CAD build for the part. Positions are in the model's coordinates, mm. A direction names the side the tool comes from. Give positions to 0.01 mm unless a question says otherwise; leave off trailing zeros. Order: outer loops, then holes, each group sorted by start corner. A loop starts at its lowest first (then second) coordinate and runs counter-clockwise, first axis right, second up. Notation, with made-up numbers: M -34.5,74.5 L -3.5,74.5 A19 ccw -3.5,107.5 Z; hole C 12,-17 d6. An arc over 180 degrees is marked long. Put each result on its own line as item: value. Start each with the question number.
1) Cut at B-B (x = -49). Write the cut outline in (y, z).
2) Cut at A-A (y = 15.5). Write the cut outline in (x, z), and give its area (3 significant figures).
3) Two-plate mould, pull along Y, no slides. Class faces 1 (the face through (-51.5, 0, 1)), 2 (the face through (-49.921, 16.345, 0.862)), 3 (the face through (11, -13.99, 5)): released by +Y, released by -Y, zero draft, split by the parting line, or undercut.
4) Tool access for faces 4 (the face through (49, 0, 4.2)), 5 (the face through (49.523, -5.072, 2.932)), 6 (the face through (49.47, 4.92, 2.93)), 7 (the face through (-23.96, -1, 5)), 8 (the face through (11, 13.01, 5)): list every direction of +Z, -Z, +X, -X, +Y, -Y with a clear straight run to the whole face (end or side of a thin tool).
5) Pin check, flat tips, straight feed: pin 1 (1.2 mm diameter, centred on x = 50, y = -1.5, fed in from +Z); pin 2 (1 mm diameter, centred on y = -14, z = 4.5, fed in from -X); pin 3 (1.5 mm diameter, centred on x = -11.5, z = 7, fed in from -Y). Stop position of each tip, or through.
6) Cut at C-C (x = -18). Write the cut outline in (y, z).
7) Drill centre lines: line 1 (Y direction, x = 49, z = 1.3); line 2 (Z direction, x = -24.5, y = 12); line 3 (Y direction, x = 1.5, z = 8.25). Where is each one in solid material? Low to high. Write a range as [from, to].
8) Cut at D-D (y = 10). Write the cut outline in (x, z), and give its area (3 significant figures).
```python
from build123d import *

# Parameters (mm, degrees)
CROQUIS1_W              = 103
CROQUIS1_H              = 36
SALIENTE_EXTRUIR1_DEPTH = 1.7
CROQUIS2_W              = 71.45
CROQUIS2_H              = 27
SALIENTE_EXTRUIR2_DEPTH = 7.05
CROQUIS3_R              = 1.25
CORTAR_EXTRUIR1_DEPTH   = 6
SALIENTE_EXTRUIR3_DEPTH = 2.5


with BuildPart() as part:
    # Croquis1 → Saliente-Extruir1 (new body)
    with BuildSketch(Plane.XY):
        Rectangle(CROQUIS1_W, CROQUIS1_H)
    extrude(amount=SALIENTE_EXTRUIR1_DEPTH)

    # Croquis2 → Saliente-Extruir2 (add)
    with BuildSketch(Plane.XY.offset(1.7)):
        with Locations((11.765, -0.49)):
            Rectangle(CROQUIS2_W, CROQUIS2_H)
    extrude(amount=SALIENTE_EXTRUIR2_DEPTH)

    # Croquis3 → Cortar-Extruir1 (cut)
    with BuildSketch(Plane.XY.offset(1.7)):
        with Locations((-49, 15.5)):
            Circle(CROQUIS3_R)
        with Locations((-49, -15.5)):
            Circle(CROQUIS3_R)
        with Locations((49, 15.5)):
            Circle(CROQUIS3_R)
        with Locations((49, -15.5)):
            Circle(CROQUIS3_R)
    extrude(amount=-CORTAR_EXTRUIR1_DEPTH, mode=Mode.SUBTRACT)

    # Croquis4 → Saliente-Extruir3 (add)
    with BuildSketch(Plane.XY.offset(1.7)):
        Polygon((47.49, 7.01), (51.5, 2.775802991), (51.5, -2.234197009), (47.49, -7.99), align=None)
    extrude(amount=SALIENTE_EXTRUIR3_DEPTH)


solid = part.part
```
Solution:
1. outline: M -18,0 L -16.75,0 L -16.75,1.7 L -18,1.7 Z; M -14.25,0 L 14.25,0 L 14.25,1.7 L -14.25,1.7 Z; M 16.75,0 L 18,0 L 18,1.7 L 16.75,1.7 Z
2. outline: M -51.5,0 L -50.25,0 L -50.25,1.7 L -51.5,1.7 Z; M -47.75,0 L 47.75,0 L 47.75,1.7 L -47.75,1.7 Z; M 50.25,0 L 51.5,0 L 51.5,1.7 L 50.25,1.7 Z
2. area: 167 mm²
3. face 1: zero draft
3. face 2: undercut
3. face 3: released by -Y
4. face 4: +Z, +X, +Y, -Y
4. face 5: +Z, +X, -Y
4. face 6: +Z, +X, +Y
4. face 7: +Z, -X, +Y, -Y
4. face 8: +Z, +X, -X, +Y
5. pin 1: z = 4.2
5. pin 2: x = -23.96
5. pin 3: y = -13.99
6. outline: M -18,0 L 18,0 L 18,1.7 L 13.01,1.7 L 13.01,8.75 L -13.99,8.75 L -13.99,1.7 L -18,1.7 Z
7. line 1: [-18, -16.75], [-14.25, 14.25], [16.75, 18]
7. line 2: [0, 1.7]
7. line 3: [-13.99, 13.01]
8. outline: M -51.5,0 L 51.5,0 L 51.5,1.7 L 47.49,1.7 L 47.49,8.75 L -23.96,8.75 L -23.96,1.7 L -51.5,1.7 Z
8. area: 679 mm²
